Drawing for the job (mm, zero at the part's lowest x, y, z). A direction names the side the tool comes from. Give positions to 0.01 mm unless a question says otherwise; leave off trailing zeros. Write each loop counter-clockwise with the first axis right and the second up, starting at its lowest first coordinate (ties: lowest second). Pieces come first, ordered by that corner, then holes. Notation, with made-up numbers: M 85,54.25 L 93,54.25 A24 cw 93,67.25 Z; hole C 31.5,-4.5 d4. An arc over 180 degrees is marked long. Use CSV: the item, a comma, the result in double quotes. Start each with the question number.
1. Mould opens along X. For the marked faces 3, 4 and 5 say: pulls with the +X half, pulls with the -X half, needs draft (parallel to the pull), parting line crosses it, or undercut.
2. Band-saw the part on A-A, the plane x = 6.05. List the corners of the cut face in (y, z) (3 decimals), then the cut area to 3 significant figures.
3. Band-saw the part on C-C, the plane z = 1. List the corners of the cut face in (x, y).
4. Band-saw the part on D-D, the plane x = 3. List the corners of the cut face in (y, z), then the cut area to 3 significant figures.
5. 3-axis set-ups, long thin cutter, end or side, ignore diameter. For the marked faces 1 and 2: which of +Z, -Z, +X, -X, +Y, -Y reach the whole face in a straight line?
6. Drill centre lines: line 1 along Y through (x, z) = (6.05, 6.75) (3 decimals); line 2 along Y through (x, z) = (6.05, 1); line 3 along X through (y, z) = (4.25, 2.75). Where is each one in solid material? Low to high. Write a range as from..to.
7. Drop flat-ended pins along their axis: pin 1 Ø1 at (x, y) = (11, 3) entering from +Z; pin 2 Ø1.5 at (x, z) = (2.5, 5.5) entering from +Y; pin 3 Ø2 at (y, z) = (10.5, 3) entering from -X. Give the stop position or say it passes through.
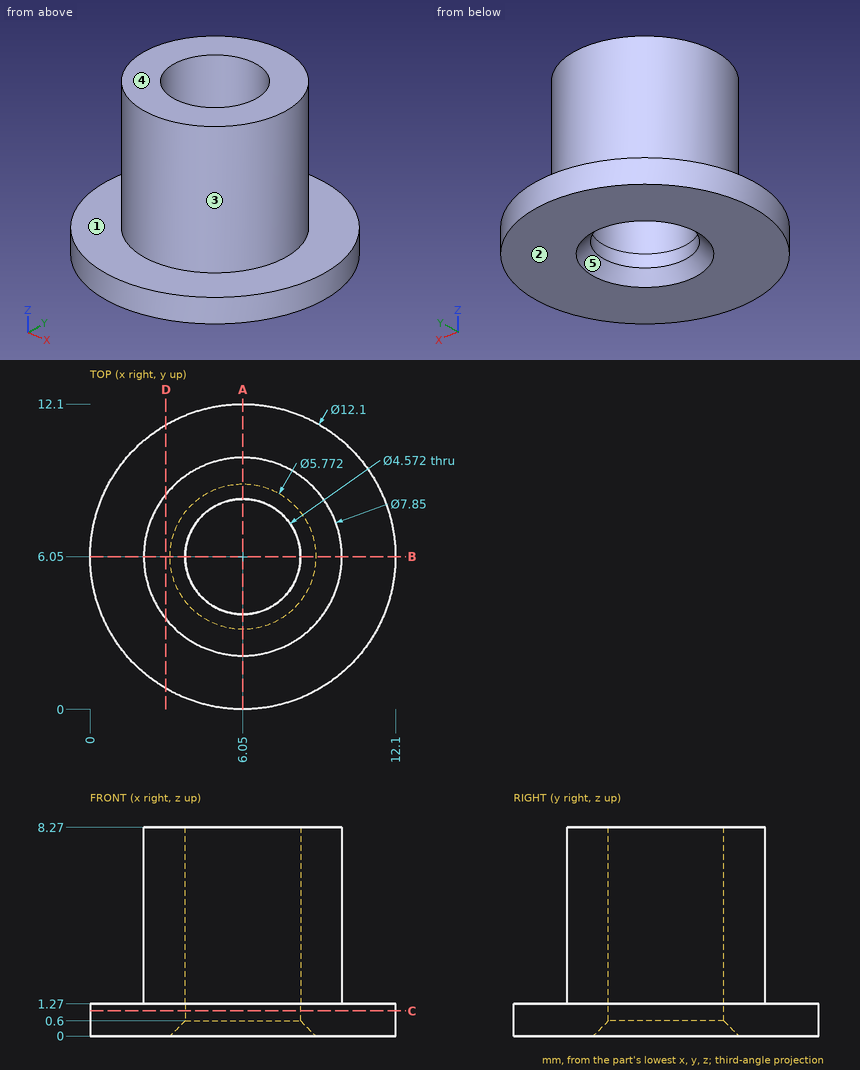
Output:
1,face 3,"parting line crosses it"
1,face 4,"needs draft"
1,face 5,"undercut"
2,outline,"M 0,0 L 3.164,0 L 3.764,0.6 L 3.764,8.27 L 2.125,8.27 L 2.125,1.27 L 0,1.27 Z; M 8.336,0.6 L 8.936,0 L 12.1,0 L 12.1,1.27 L 9.975,1.27 L 9.975,8.27 L 8.336,8.27 Z"
2,area,"32.1 mm²"
3,outline,"C 6.05,6.05 d12.1; hole C 6.05,6.05 d4.57"
4,outline,"M 0.83,0 L 11.27,0 L 11.27,1.27 L 8.52,1.27 L 8.52,8.27 L 3.58,8.27 L 3.58,1.27 L 0.83,1.27 Z"
4,area,"47.9 mm²"
5,face 1,"+Z"
5,face 2,"-Z, +X, -X, +Y, -Y"
6,line 1,"y = 2.125..3.764, 8.336..9.975"
6,line 2,"y = 0..3.76, 8.34..12.1"
6,line 3,"x = 2.56..4.64, 7.46..9.54"
7,pin 1,"stops at z = 1.27"
7,pin 2,"stops at y = 8.8"
7,pin 3,"stops at x = 4.18"
